```python
from build123d import *

# Parameters (mm, degrees)
F0_W     = 84.3321233988
F0_H     = 88.7495167553
F1_DEPTH = 76.2
F4_W     = 28.8745099679
F4_H     = 1.0582283139
F5_DEPTH = 0.254
F7_W     = 16.5562033653
F7_H     = 1.3796836138
F8_DEPTH = 2.54


# Not quite as in the source:
# - the program builds the solid bodies; features that only make, move or delete a surface that nothing else refers to are left out


with BuildPart() as f1:
    # F0 (on Top) → F1 (new body)
    with BuildSketch(Plane.XY):
        with Locations((4.1730180383, -8.0741699785)):
            Rectangle(F0_W, F0_H)
    extrude(amount=F1_DEPTH)

    # F4 (on face) → F5 (join)
    with BuildSketch(Plane.XZ.offset(52.4489283562)):
        with Locations((-1.3617197983, 52.3322783411)):
            Rectangle(F4_W, F4_H)
        Polygon((13.0755351856, 55.5825531483), (13.0755351856, 52.861392498), (13.0755351856, 51.8031641841), (13.0755351856, 49.0820072591), (18.8202019781, 51.8031641841), align=None)
    extrude(amount=F5_DEPTH)

    # F7 (on offset) → F8 (join)
    with BuildSketch(Plane(origin=(28.8089563389, 0, 0), x_dir=(0, -1, 0), z_dir=(-1, 0, 0))):
        with Locations((54.5372888446, 35.6855541468)):
            Rectangle(F7_W, F7_H)
        Polygon((62.8153905272, 39.0911102295), (62.8153905272, 36.3753959537), (62.8153905272, 34.9957123399), (62.8153905272, 32.7537246048), (67.8167492151, 36.3753959537), align=None)
    extrude(amount=F8_DEPTH)


solid = f1.part
```
Check sheet for the modelled part. Datum: model origin and axes. Units: mm. A direction names the side the tool comes from. Round coordinates to 2 decimals unless told otherwise and drop trailing zeros. Loops run counter-clockwise (first coordinate to the right, second up) from the corner with the lowest first, then second, coordinate; pieces in that order, holes last. Notation, with made-up numbers: (48.25, 7.5) -> (73.25, 7.5) arc R25 ccw to (73.25, 26.5) -> close; hole circle Ø6 at (60, -30). An arc over 180 degrees is marked (long way). Answer in a Markdown table with one row per item.
Q1. Go/stop test with flat-tipped pins: P1, Ø23, axis at x = 5, z = 33.5, coming from the -Y side; P2, Ø1.9, axis at y = -61, z = 36.5, coming from the +X side; P3, Ø2, axis at x = 27, y = -57.5, coming from the -Z side; P4, Ø4, axis at x = 15.5, y = -13.5, coming from the -Z side. Record where each tip stops, or that it passes through.
Data:
| item | result |
|---|---|
| P1 | stops at y = -52.45 |
| P2 | stops at x = 28.81 |
| P3 | stops at z = 35 |
| P4 | stops at z = 0 |
Q2. Sectioned sample at B-B on z = 44.5. Enter the section's corners in (x, y), then the cut area to 3 significant figures.
Data:
| item | result |
|---|---|
| outline | (-37.99, -52.45) -> (46.34, -52.45) -> (46.34, 36.3) -> (-37.99, 36.3) -> close |
| area | 7,480 mm^2 |
Q3. Sectioned sample at A-A on x = 8.5. Enter the section's corners in (y, z).
Data:
| item | result |
|---|---|
| outline | (-52.7, 51.8) -> (-52.45, 51.8) -> (-52.45, 0) -> (36.3, 0) -> (36.3, 76.2) -> (-52.45, 76.2) -> (-52.45, 52.86) -> (-52.7, 52.86) -> close |
Q4. Set-up check for faces 1 (the face through (28.809, -61, 36)), 2 (the face through (26.269, -61, 36)), 3 (the face through (-37.993, -9, 38)), 4 (the face through (28, -62.815, 38)), 5 (the face through (27.56, -65.28, 34.54)): record each of +Z, -Z, +X, -X, +Y, -Y from which the full face is reachable in a straight line by a thin tool's end or side.
Data:
| item | result |
|---|---|
| face 1 | +Z, -Z, +X, -Y |
| face 2 | +Z, -Z, -X, -Y |
| face 3 | +Z, -Z, -X, +Y, -Y |
| face 4 | +Z, +X, -X |
| face 5 | -Z, +X, -X, -Y |
Q5. Thickness scan on L1, parallel to Y at x = -10, z = 55. Record the ranges inside material, lowest first.
Data:
| item | result |
|---|---|
| L1 | y = -52.45 to 36.3 |
Q6. Release check for a two-part mould opening along Y. For faces 6 (the face through (27.557, -65.351, 37.714)), 7 (the face through (28, -58, 34.996)), 8 (the face through (46.339, -9, 38)), 9 (the face through (28, -58, 36.375)) record: released by +Y, released by -Y, zero draft, split by the parting line, or undercut.
Data:
| item | result |
|---|---|
| face 6 | released by -Y |
| face 7 | undercut |
| face 8 | zero draft |
| face 9 | undercut |
Q7. Sectioned sample at C-C on x = 24. Enter the section's corners in (y, z).
Data:
| item | result |
|---|---|
| outline | (-52.45, 0) -> (36.3, 0) -> (36.3, 76.2) -> (-52.45, 76.2) -> close |
